from build123d import *

# Parameters (mm, degrees)
ESQUISSE1_R             = 13
BOSS_EXTRU_1_DEPTH      = 44.7
ESQUISSE2_R             = 4
BOSS_EXTRU_2_DEPTH      = 1
ESQUISSE3_R             = 1.5
BOSS_EXTRU_3_DEPTH      = 10
ENL_V_START             = -7
ENL_V_MAT_EXTRU_1_DEPTH = 7


with BuildPart() as part:
    # Esquisse1 → Boss.-Extru.1 (new body)
    with BuildSketch(Plane.XY):
        with Locations(Location((0, 0, 0), (0, 0, 180))):
            Circle(ESQUISSE1_R)
    extrude(amount=BOSS_EXTRU_1_DEPTH)

    # Esquisse2 → Boss.-Extru.2 (add)
    with BuildSketch(Plane.XY.offset(44.7)):
        Circle(ESQUISSE2_R)
    extrude(amount=BOSS_EXTRU_2_DEPTH)

    # Esquisse3 → Boss.-Extru.3 (add)
    with BuildSketch(Plane.XY.offset(45.7)):
        Circle(ESQUISSE3_R)
    extrude(amount=BOSS_EXTRU_3_DEPTH)

    # Esquisse4 → Enlèv. mat.-Extru.1 (cut)
    with BuildSketch(Plane.XY.offset(55.7).offset(ENL_V_START)):
        with BuildLine():
            Line((-1.200903118, 0.898794582), (1.200903118, 0.898794582))
            ThreePointArc((1.200903118, 0.898794582), (0, 1.5), (-1.200903118, 0.898794582))
        make_face()
    extrude(amount=ENL_V_MAT_EXTRU_1_DEPTH, mode=Mode.SUBTRACT)


solid = part.part
Could you check a few things on this model? Use its own coordinates, in mm. A direction names the side the tool comes from. Give positions to 0.01 mm unless a question says otherwise; leave off trailing zeros. Order: outer loops, then holes, each group sorted by start corner. A loop starts at its lowest first (then second) coordinate and runs counter-clockwise, first axis right, second up. Notation, with made-up numbers: (27.25, -39) -> (35.25, -39) arc R22 cw to (35.25, -4) -> close; hole circle Ø9 at (4, 64). An arc over 180 degrees is marked (long way). Answer in a Markdown table with one row per item. Add a question column.
Item 1: I'm going to push flat-ended pins straight in: P1, Ø3, axis at x = -10, z = 45, coming from the -Y side; P2, Ø0.5, axis at x = 0, y = 1.5, coming from the +Z side; P3, Ø1, axis at y = 4, z = 40, coming from the +X side. Where does each tip first touch, or does it pass through?
Item 2: Imagine slicing it at A-A (y = 0). List the corners of the cut face in (x, z) for me.
Item 3: Imagine slicing it at D-D (x = -3.25). List the corners of the cut face in (y, z) for me, and give its area (3 significant figures).
Item 4: Imagine slicing it at C-C (z = 40). List the corners of the cut face in (x, y) for me, and give its area (3 significant figures).
Item 5: Imagine slicing it at B-B (x = 0). List the corners of the cut face in (y, z) for me.
Item 6: For faces 1 (the flat face through (2, 0, 45.7)), 2 (the flat face through (0, 0, 55.7)), 3 (the flat face through (0, 0.899, 52)), which set-ups out of +Z, -Z, +X, -X, +Y, -Y let a thin tool reach every point of the face, with its end or its side?
Item 7: Please list where these lines run through material, in increasing order: probe 1 along Z at (x, y) = (-5, 10.5); probe 2 along X at (y, z) = (-7.25, 13.5); probe 3 along X at (y, z) = (0, 52.5).
Result:
| question | item | result |
|---|---|---|
| 1 | P1 | y = -9.81 |
| 1 | P2 | z = 48.7 |
| 1 | P3 | x = 12.52 |
| 2 | outline | (-13, 0) -> (13, 0) -> (13, 44.7) -> (4, 44.7) -> (4, 45.7) -> (1.5, 45.7) -> (1.5, 55.7) -> (-1.5, 55.7) -> (-1.5, 45.7) -> (-4, 45.7) -> (-4, 44.7) -> (-13, 44.7) -> close |
| 3 | outline | (-12.59, 0) -> (12.59, 0) -> (12.59, 44.7) -> (2.33, 44.7) -> (2.33, 45.7) -> (-2.33, 45.7) -> (-2.33, 44.7) -> (-12.59, 44.7) -> close |
| 3 | area | 1,130 mm2 |
| 4 | outline | circle Ø26 at (0, 0) |
| 4 | area | 531 mm2 |
| 5 | outline | (-13, 0) -> (13, 0) -> (13, 44.7) -> (4, 44.7) -> (4, 45.7) -> (1.5, 45.7) -> (1.5, 48.7) -> (0.9, 48.7) -> (0.9, 55.7) -> (-1.5, 55.7) -> (-1.5, 45.7) -> (-4, 45.7) -> (-4, 44.7) -> (-13, 44.7) -> close |
| 6 | face 1 | +Z |
| 6 | face 2 | +Z, +X, -X, +Y, -Y |
| 6 | face 3 | +Z, +X, -X, +Y |
| 7 | probe 1 | 0 to 44.7 |
| 7 | probe 2 | -10.79 to 10.79 |
| 7 | probe 3 | -1.5 to 1.5 |
